from build123d import *

# Parameters (mm, degrees)
CHAMFER1_SIZE      = 0.3
SKETCH2_W          = 2.25
SKETCH2_H          = 2.25
CUT_EXTRUDE1_DEPTH = 30


with BuildPart() as part:
    # Sketch1 → Revolve1 (revolve)
    with BuildSketch(Plane.XY, mode=Mode.PRIVATE) as revolve1_sk:
        Polygon((0, 0), (4, 0), (4, 30), (5, 30), (5, 90), (0, 90), align=None)
    revolve(revolve1_sk.sketch.rotate(Axis((0, 90, 0), (0, -1, 0)), 180), axis=Axis((0, 90, 0), (0, -1, 0)))

    # Chamfer1
    chamfer1_edges = [part.edges().sort_by_distance(p)[0] for p in [
        (4, 0, 0),
    ]]
    chamfer(chamfer1_edges, length=CHAMFER1_SIZE)

    # Sketch2 → Cut-Extrude1 (cut)
    with BuildSketch(Plane.XZ):
        with Locations((0, 4)):
            Rectangle(SKETCH2_W, SKETCH2_H)
    extrude(amount=-CUT_EXTRUDE1_DEPTH, mode=Mode.SUBTRACT)


solid = part.part
Work out the finished part from the listing and answer in its coordinate system (mm). Coordinates: 2 decimals unless noted, no trailing zeros. Write each loop counter-clockwise with the first axis right and the second up, starting at its lowest first coordinate (ties: lowest second). Pieces come first, ordered by that corner, then holes. Notation, with made-up numbers: M 83,0 L 110,0 A33 cw 110,33 Z; hole C 75.5,17.25 d6. An arc over 180 degrees is marked long. Use one line per item in the form item = value. Start each with the question number.
1. Straight lines are drawn through the part: probe 1 along Z at (x, y) = (3, 48.5); probe 2 along Z at (x, y) = (-0.25, 67); probe 3 along Y at (x, z) = (2.5, -3.5). For each, find the intervals that lie inside material, in ascending order. Write a range as from..to.
2. The part is cut by section B-B (x = 0). Give the vertices of the cut face in (y, z) (3 decimals).
3. The part is cut by section C-C (y = 61.5). Give the vertices of the cut face in (x, z), plus the area to 3 significant figures.
4. Each of these flat-tipped pins is pushed along its axis until it touches: P1, Ø1.8, axis at x = -0.5, y = 9, coming from the +Z side; P2, Ø1.5, axis at x = 2, y = 28.5, coming from the -Z side; P3, Ø0.5, axis at y = 20, z = 3, coming from the -X side. Where does it stop, or does it pass through?
5. The part is cut by section A-A (z = 0). Give the vertices of the cut face in (x, y), plus the area to 3 significant figures.
6. The mould has two halves that part along X. Classify faces 1 (the face through (0, 90, 0)), 2 (the face through (0, 15, -4)), 3 (the face through (0, 15, 2.875)): released by +X, released by -X, zero draft, split by the parting line, or undercut.
Evaluation:
q1.probe_1 = -4..4
q1.probe_2 = -4.99..4.99
q1.probe_3 = 30..90
q2.outline = M 0,-3.7 L 0.3,-4 L 30,-4 L 30,-5 L 90,-5 L 90,5 L 30,5 L 30,2.875 L 0,2.875 Z
q3.outline = C 0,0 d10
q3.area = 78.5 mm^2
q4.P1 = 3.84
q4.P2 = -3.8
q4.P3 = -2.9
q5.outline = M -5,30 L -4,30 L -4,0.3 L -3.7,0 L 3.7,0 L 4,0.3 L 4,30 L 5,30 L 5,90 L -5,90 Z
q5.area = 840 mm^2
q6.face_1 = zero draft
q6.face_2 = split by the parting line
q6.face_3 = undercut
